Model file for the job. Use its own axes, mm. A direction names the side the tool comes from. Round coordinates to 2 decimals unless told otherwise and drop trailing zeros. Loops run counter-clockwise (first coordinate to the right, second up) from the corner with the lowest first, then second, coordinate; pieces in that order, holes last.
from build123d import *

# Parameters (mm, degrees)
SKETCH2_W           = 40
SKETCH2_H           = 13
BOSS_EXTRUDE1_DEPTH = 3
SKETCH3_W           = 3
SKETCH3_H           = 13
BOSS_EXTRUDE2_DEPTH = 10
SKETCH4_R           = 2
CUT_EXTRUDE1_DEPTH  = 12
CUT_EXTRUDE2_DEPTH  = 12


with BuildPart() as part:
    # Sketch2 → Boss-Extrude1 (new body)
    with BuildSketch(Plane.XY):
        Rectangle(SKETCH2_W, SKETCH2_H)
    extrude(amount=BOSS_EXTRUDE1_DEPTH)

    # Sketch3 → Boss-Extrude2 (add)
    with BuildSketch(Plane.XY.offset(3)):
        with Locations((-18.5, 0)):
            Rectangle(SKETCH3_W, SKETCH3_H)
    extrude(amount=BOSS_EXTRUDE2_DEPTH)

    # Sketch4 → Cut-Extrude1 (cut)
    with BuildSketch(Plane.ZY.offset(20)):
        with Locations((6.5, 0)):
            Circle(SKETCH4_R)
    extrude(amount=-CUT_EXTRUDE1_DEPTH, mode=Mode.SUBTRACT)

    # Sketch5 → Cut-Extrude2 (cut)
    with BuildSketch(Plane(origin=(0, 0, 0), x_dir=(-1, 0, 0), z_dir=(0, 0, -1))):
        with BuildLine():
            Line((-15, 2), (11.584611172, 2))
            ThreePointArc((11.584611172, 2), (13.584611172, 0), (11.584611172, -2))
            Line((11.584611172, -2), (-15, -2))
            ThreePointArc((-15, -2), (-17, 0), (-15, 2))
        make_face()
    extrude(amount=-CUT_EXTRUDE2_DEPTH, mode=Mode.SUBTRACT)


solid = part.part
Q1. Probe line 1 (Y direction, x = -0.5, z = 1.75); line 2 (X direction, y = 1, z = 11.25); line 3 (Z direction, x = -6.5, y = -4). List the from-to ranges inside material, lowest first.
Q2. Slice it at D-D on y = -2.5. Give the cut face in (x, z).
Q3. Slice it at C-C on y = 0. Give the cut face in (x, z).
Q4. Tool access for faces 1 (the face through (17, 0, 1)), 2 (the face through (-19, 0, 13)), 3 (the face through (1, 3, 3)): list every direction of +Z, -Z, +X, -X, +Y, -Y with a clear straight run to the whole face (end or side of a thin tool).
Q5. Pull direction Y, two halves, no side cores. Call faces 4 (the face through (0, 3, 0)), 5 (the face through (-4.5, -6.5, 2.6)), 6 (the face through (-13.584, 0.044, 1.479)): pulls with the +Y half, pulls with the -Y half, needs draft (parallel to the pull), parting line crosses it, or undercut.
Q6. Flat gauge pins, fed straight in: P1, Ø3, axis at y = 0, z = 6.5, coming from the +X side; P2, Ø1, axis at x = 5, y = 2.5, coming from the -Z side; P3, Ø4, axis at x = -5.5, y = 2.5, coming from the +Z side. Where does each tip first touch, or does it go through?
Q7. Slice it at B-B on z = 6.5. Give the cut face in (x, y).
Q8. Slice it at A-A on x = 0. Give the cut face in (y, z).
Reply:
1. line 1: y = -6.5 to -2, 2 to 6.5
1. line 2: x = -20 to -17
1. line 3: z = 0 to 3
2. outline: (-20, 0) - (20, 0) - (20, 3) - (-17, 3) - (-17, 13) - (-20, 13) - close
3. outline: (-20, 0) - (-13.58, 0) - (-13.58, 3) - (-17, 3) - (-17, 4.5) - (-20, 4.5) - close; (-20, 8.5) - (-17, 8.5) - (-17, 13) - (-20, 13) - close; (17, 0) - (20, 0) - (20, 3) - (17, 3) - close
4. face 1: +Z, -Z
4. face 2: +Z, +X, -X, +Y, -Y
4. face 3: +Z, +X, +Y, -Y
5. face 4: needs draft
5. face 5: pulls with the -Y half
5. face 6: undercut
6. P1: passes through
6. P2: stops at z = 0
6. P3: stops at z = 3
7. outline: (-20, -6.5) - (-17, -6.5) - (-17, -2) - (-20, -2) - close; (-20, 2) - (-17, 2) - (-17, 6.5) - (-20, 6.5) - close
8. outline: (-6.5, 0) - (-2, 0) - (-2, 3) - (-6.5, 3) - close; (2, 0) - (6.5, 0) - (6.5, 3) - (2, 3) - close
